Verification items for the finished model (mm, model axes). Face numbers are marked on the shaded views. A direction names the side the tool comes from. Coordinates: 2 decimals unless noted, no trailing zeros. Order: outer loops, then holes, each group sorted by start corner. A loop starts at its lowest first (then second) coordinate and runs counter-clockwise, first axis right, second up. Notation, with made-up numbers: (-29.75, 20) - (-6.75, 20) arc R15 cw to (-6.75, 24) - close; hole circle Ø6 at (31, 84.5). An arc over 180 degrees is marked (long way). One line per question, with ' | ' between items. Start each with the question number.
Autodesk Inventor part; units mm, degrees
ref_plane "YZ Plane" through (0, 0, 0) normal (1, 0, 0) x (0, 1, 0)
ref_plane "XZ Plane" through (0, 0, 0) normal (0, 1, 0) x (-1, 0, 0)
ref_plane "XY Plane" through (0, 0, 0) normal (0, 0, 1) x (1, 0, 0)
sketch "Skizze1" plane through (0, 0, 0) normal (0, 0, 1) x (1, 0, 0)
  line L0 (-10, -20.3) -> (10, -20.3)
  line L1 (10, -20.3) -> (10, 20.3)
  line L2 (10, 20.3) -> (-10, 20.3)
  line L3 (-10, 20.3) -> (-10, -20.3)
  line L4 (-10, -20.3) -> (10, 20.3) construction
  line L5 (10, -20.3) -> (-10, 20.3) construction
  point P0 (0, 0)
  dimension "d0" = 20
  dimension "d1" = 40.6
extrude "Extrusion1" add sketch "Skizze1" along normal blind 26.5
sketch "Skizze2" plane through (0, 0, 26.5) normal (0, 0, 1) x (1, 0, 0)
  point P0 (0, 0)
sketch "Skizze3" plane through (0, 0, 26.5) normal (0, 0, 1) x (1, 0, 0)
  line L0 (-10, 20.3) -> (-10, -20.3)
  line L1 (10, -20.3) -> (10, 20.3)
  line L2 (10, 20.3) -> (-10, 20.3)
  line L3 (-10, -20.3) -> (10, -20.3)
  line L4 (-10, -27.25) -> (10, -27.25)
  line L5 (10, -27.25) -> (10, 27.25)
  line L6 (10, 27.25) -> (-10, 27.25)
  line L7 (-10, 27.25) -> (-10, -27.25)
  line L8 (-10, -27.25) -> (10, 27.25) construction
  line L9 (10, -27.25) -> (-10, 27.25) construction
  point P0 (0, 0)
  dimension "d4" = 54.5
  dimension "d5" = 0
extrude "Extrusion2" add sketch "Skizze3" along normal blind 2.5
sketch "Skizze4" plane through (0, 0, 29) normal (0, 0, 1) x (1, 0, 0)
  line L0 (10, -20.3) -> (10, 20.3)
  line L1 (-10, -20.3) -> (10, -20.3)
  line L2 (10, -20.3) -> (10, 20.3)
  line L3 (10, 20.3) -> (-10, 20.3)
  line L4 (-10, 20.3) -> (-10, -20.3)
  line L5 (-10, -20.3) -> (10, 20.3) construction
  line L6 (10, -20.3) -> (-10, 20.3) construction
  point P0 (0, 0)
  dimension "d8" = 40.6
extrude "Extrusion3" add sketch "Skizze4" along normal blind 9.9
sketch "Skizze6" plane through (0, 0, 29) normal (0, 0, 1) x (1, 0, 0)
  line L0 (10, -27.25) -> (-10, -27.25)
  line L1 (-10, -27.25) -> (-10, -20.3)
  line L2 (10, -20.3) -> (-10, -20.3)
  line L3 (10, 20.3) -> (10, -20.3)
  line L4 (-10, 20.3) -> (10, 20.3)
  line L5 (-10, 20.3) -> (-10, 27.25)
  line L6 (-10, 27.25) -> (10, 27.25)
  line L7 (10, 27.25) -> (10, 20.3)
  line L8 (10, -20.3) -> (10, -27.25)
  line L9 (-10, -20.3) -> (-10, 20.3)
  circle A0 centre (5, 24.75) radius 2.25
  line L10 (-14, 0) -> (14, 0)
  line L11 (0, 38.15) -> (0, -38.15)
  point P0 (0, 0)
  dimension "d12" = 24.75
  dimension "d13" = 5
  dimension "d14" = 4.5
extrude "Extrusion4" cut sketch "Skizze6" against normal blind 9.9 contours A0
mirror "Spiegeln1" about plane through (0, 0, 0) normal (0, 1, 0) of "Extrusion4"
mirror "Spiegeln2" about plane through (0, 0, 0) normal (1, 0, 0) of "Extrusion4", "Spiegeln1"
sketch "Skizze7" plane through (0, 0, 38.9) normal (0, 0, 1) x (1, 0, 0)
  line L0 (0, 38.15) -> (0, -38.15)
  line L1 (-14, 0) -> (14, 0)
  circle A0 centre (-5, -24.75) radius 2.25
  circle A1 centre (5, -24.75) radius 2.25
  circle A2 centre (0, -9.9) radius 2.5
  point P0 (0, 0)
  dimension "d18" = 14.85
  dimension "d19" = 5
extrude "Extrusion5" add sketch "Skizze7" along normal blind 5 contours A2 L0 | L0 A2
chamfer "Fase1" distance 2 angle 45 4 edges at (0, -20.3, 38.9) (0, 20.3, 38.9) (10, 0, 38.9) (-10, 0, 38.9)
properties part number "Servo_Drehwerk" material "Aluminium 6061"
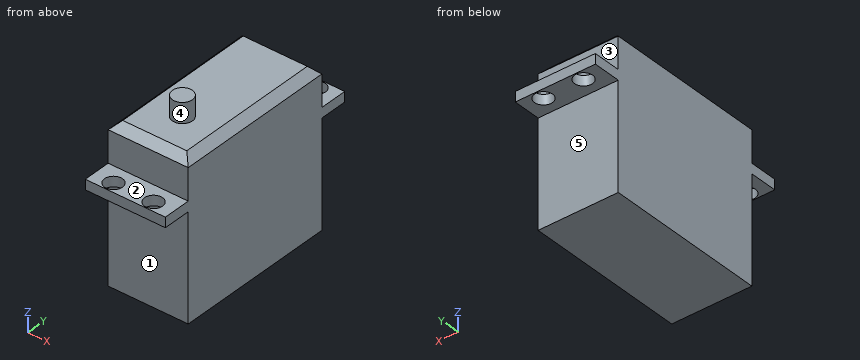
Item 1: Thickness scan on probe 1 along X at (y, z) = (-24.75, 27.8); probe 2 along Z at (x, y) = (1.5, 5.5); probe 3 along Y at (x, z) = (6.5, 33.5). Record the ranges inside material, lowest first. Write a range as from..to.
Item 2: Set-up check for the marked faces 1, 2, 3, 4 and 5: record each of +Z, -Z, +X, -X, +Y, -Y from which the full face is reachable in a straight line by a thin tool's end or side.
Item 3: Section check C-C (x = -1.5). Record the cut outline in (y, z).
Item 4: Section check D-D (y = -9.9). Record the cut outline in (x, z), then the cut area to 3 significant figures.
Item 5: Section check A-A (x = 5). Record the cut outline in (y, z).
Item 6: Section check B-B (y = 24.75). Record the cut outline in (x, z), then the cut area to 3 significant figures.
Item 7: Gauge pin test, flat ends, axial feed: pin 1 (5.5 mm diameter, centred on x = 1.5, y = 22, fed in from +Z); pin 2 (2 mm diameter, centred on x = -6.5, z = 8, fed in from +Y); pin 3 (1 mm diameter, centred on y = 11.5, z = 38, fed in from -X). Record the tip position at first contact, or that the pin passes through.
Completed:
1) probe 1: x = -10..-7.25, -2.75..2.75, 7.25..10 | probe 2: z = 0..38.9 | probe 3: y = -20.3..20.3
2) face 1: -Z, +X, -X, -Y | face 2: +Z, +X, -X, -Y | face 3: +Z, +X, -X, +Y | face 4: +Z | face 5: -Z, +X, -X, +Y
3) outline: (-27.25, 26.5) - (-20.3, 26.5) - (-20.3, 0) - (20.3, 0) - (20.3, 26.5) - (27.25, 26.5) - (27.25, 29) - (20.3, 29) - (20.3, 36.9) - (18.3, 38.9) - (-7.9, 38.9) - (-7.9, 43.9) - (-11.9, 43.9) - (-11.9, 38.9) - (-18.3, 38.9) - (-20.3, 36.9) - (-20.3, 29) - (-27.25, 29) - close
4) outline: (-10, 0) - (10, 0) - (10, 36.9) - (8, 38.9) - (2.5, 38.9) - (2.5, 43.9) - (-2.5, 43.9) - (-2.5, 38.9) - (-8, 38.9) - (-10, 36.9) - close | area: 799 mm^2
5) outline: (-27.25, 26.5) - (-27, 26.5) - (-27, 29) - (-27.25, 29) - close; (-22.5, 26.5) - (-20.3, 26.5) - (-20.3, 0) - (20.3, 0) - (20.3, 26.5) - (22.5, 26.5) - (22.5, 29) - (20.3, 29) - (20.3, 36.9) - (18.3, 38.9) - (-18.3, 38.9) - (-20.3, 36.9) - (-20.3, 29) - (-22.5, 29) - close; (27, 26.5) - (27.25, 26.5) - (27.25, 29) - (27, 29) - close
6) outline: (-10, 26.5) - (-7.25, 26.5) - (-7.25, 29) - (-10, 29) - close; (-2.75, 26.5) - (2.75, 26.5) - (2.75, 29) - (-2.75, 29) - close; (7.25, 26.5) - (10, 26.5) - (10, 29) - (7.25, 29) - close | area: 27.5 mm^2
7) pin 1: stops at z = 37.95 | pin 2: stops at y = 20.3 | pin 3: stops at x = -9.4
